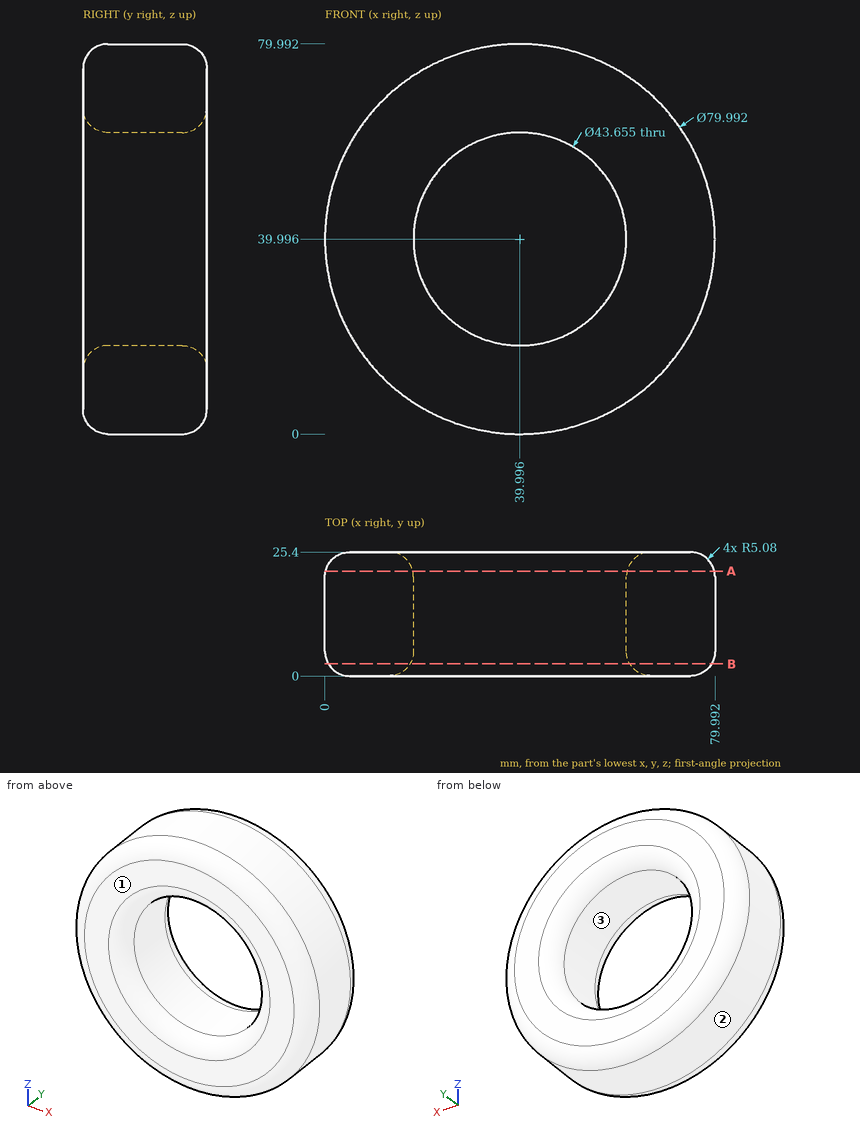
For this review, use the dimensioned drawing (mm, ordinates from the lowest corner) and the shaded views. Coordinates: 2 decimals unless noted, no trailing zeros. Write each loop counter-clockwise with the first axis right and the second up, starting at its lowest first coordinate (ties: lowest second). Pieces come first, ordered by that corner, then holes. Notation, with made-up numbers: (-0.75, 2) -> (31.25, 2) arc R21 cw to (31.25, 12) -> close; hole circle Ø1 at (41.25, 53). An arc over 180 degrees is marked (long way). Write each question's results on one line, items separated by ' | '. Start each with the question number.
(1) The part is to be moulded in two halves that separate along X. For the marked faces 1, 2 and 3, say which applies: pulls with the +X half, pulls with the -X half, needs draft (parallel to the pull), parting line crosses it, or undercut.
(2) Clearance check with flat-ended pins moving along their axes: P1, Ø10, axis at x = 58, y = 14, coming from the -Z side; P2, Ø2, axis at y = 12.5, z = 15.5, coming from the +X side; P3, Ø10, axis at x = 20.5, y = 14, coming from the -Z side. State where each tip first meets the part, or that it passes through.
(3) Take a section at B-B on y = 2.5. Write out the cut boundary in (x, z) (1 decimal).
(4) Take a section at A-A on y = 21.5. Write out the cut boundary in (x, z) (1 decimal).
(5) For line 1 along X through (y, z) = (23, 47) (1 decimal); line 2 along X through (y, z) = (4.5, 57) (1 decimal); line 3 along Z through (x, y) = (38, 22.75) (1 decimal), list the stretches that pass through material, from the lowest coordinate up. Write a range as from..to.
Results found:
1) face 1: needs draft | face 2: parting line crosses it | face 3: undercut
2) P1: stops at z = 2.17 | P2: stops at x = 72.36 | P3: stops at z = 2.72
3) outline: circle Ø78.6 at (40, 40); hole circle Ø45.1 at (40, 40)
4) outline: circle Ø79.7 at (40, 40); hole circle Ø43.9 at (40, 40)
5) line 1: x = 1.4..18.5, 61.5..78.6 | line 2: x = 3.8..26.3, 53.7..76.2 | line 3: z = 0.7..17.6, 62.4..79.3
